from build123d import *

# Parameters (mm, degrees)
SKETCH1_W           = 124.5
SKETCH1_H           = 65.5
BOSS_EXTRUDE1_DEPTH = 1
SKETCH2_R           = 3.5
BOSS_EXTRUDE2_DEPTH = 3.5
SKETCH3_R           = 1.25
BOSS_EXTRUDE3_DEPTH = 3


with BuildPart() as part:
    # Sketch1 → Boss-Extrude1 (new body)
    with BuildSketch(Plane.XY):
        Rectangle(SKETCH1_W, SKETCH1_H)
    extrude(amount=BOSS_EXTRUDE1_DEPTH)

    # Sketch2 → Boss-Extrude2 (add)
    with BuildSketch(Plane.XY.offset(1)):
        with Locations(Location((-55.75, 24.5, 0), (0, 0, 180))):
            Circle(SKETCH2_R)
        with Locations(Location((2.25, 24.5, 0), (0, 0, 180))):
            Circle(SKETCH2_R)
        with Locations(Location((2.25, -24.5, 0), (0, 0, 180))):
            Circle(SKETCH2_R)
        with Locations(Location((-55.75, -24.5, 0), (0, 0, 180))):
            Circle(SKETCH2_R)
    extrude(amount=BOSS_EXTRUDE2_DEPTH)

    # Sketch3 → Boss-Extrude3 (add)
    with BuildSketch(Plane.XY.offset(4.5)):
        with Locations((-55.75, 24.5)):
            Circle(SKETCH3_R)
        with Locations((2.25, 24.5)):
            Circle(SKETCH3_R)
        with Locations((2.25, -24.5)):
            Circle(SKETCH3_R)
        with Locations((-55.75, -24.5)):
            Circle(SKETCH3_R)
    extrude(amount=BOSS_EXTRUDE3_DEPTH)


solid = part.part
Input: part model. Units: mm. Frame: model coordinates. A direction names the side the tool comes from. Give positions to 0.01 mm unless a question says otherwise; leave off trailing zeros. Write each loop counter-clockwise with the first axis right and the second up, starting at its lowest first coordinate (ties: lowest second). Pieces come first, ordered by that corner, then holes.
Q1. Section A-A, the plane y = 24.5. Output: boundary loops of the cut face in (x, z), plus the area to 4 significant figures.
Q2. Section B-B, the plane x = -55.75. Output: boundary loops of the cut face in (y, z), plus the area to 4 significant figures.
Q3. Set-up query: faces 1 (the face through (0.37, -27.45, 2.73)), 2 (the face through (2, 25, 7.5)). Return all of +Z, -Z, +X, -X, +Y, -Y with unobstructed straight access to the full face (end or side cutting, diameter ignored); none if empty.
Q4. Pull-direction query (X, two-part tool) for faces 3 (the face through (-56, -24, 7.5)), 4 (the face through (-52.253, 24.346, 2.726)); classes: pulls with the +X half, pulls with the -X half, needs draft (parallel to the pull), parting line crosses it, or undercut.
Q5. Section C-C, the plane x = 47. Output: boundary loops of the cut face in (y, z), plus the area to 3 significant figures.
Q6. First-contact query: P1, Ø1.5, axis at y = 22, z = 4.5, coming from the -X side. Flat tip, straight axial feed; report the tip coordinate or a pass-through.
Q7. Material intervals for probe 1 along Z at (x, y) = (-40, 30.5); probe 2 along X at (y, z) = (26.5, 4); probe 3 along X at (y, z) = (-22, 1.25), sorted ascending.
Q8. Section D-D, the plane y = -5.5. Output: boundary loops of the cut face in (x, z).
Filled in:
1. outline: (-62.25, 0) - (62.25, 0) - (62.25, 1) - (5.75, 1) - (5.75, 4.5) - (3.5, 4.5) - (3.5, 7.5) - (1, 7.5) - (1, 4.5) - (-1.25, 4.5) - (-1.25, 1) - (-52.25, 1) - (-52.25, 4.5) - (-54.5, 4.5) - (-54.5, 7.5) - (-57, 7.5) - (-57, 4.5) - (-59.25, 4.5) - (-59.25, 1) - (-62.25, 1) - close
1. area: 188.5 mm2
2. outline: (-32.75, 0) - (32.75, 0) - (32.75, 1) - (28, 1) - (28, 4.5) - (25.75, 4.5) - (25.75, 7.5) - (23.25, 7.5) - (23.25, 4.5) - (21, 4.5) - (21, 1) - (-21, 1) - (-21, 4.5) - (-23.25, 4.5) - (-23.25, 7.5) - (-25.75, 7.5) - (-25.75, 4.5) - (-28, 4.5) - (-28, 1) - (-32.75, 1) - close
2. area: 129.5 mm2
3. face 1: +Z
3. face 2: +Z, +X, -X, +Y, -Y
4. face 3: needs draft
4. face 4: undercut
5. outline: (-32.75, 0) - (32.75, 0) - (32.75, 1) - (-32.75, 1) - close
5. area: 65.5 mm2
6. P1: stops at x = -58.78
7. probe 1: z = 0 to 1
7. probe 2: x = -58.62 to -52.88, -0.62 to 5.12
7. probe 3: x = -58.2 to -53.3, -0.2 to 4.7
8. outline: (-62.25, 0) - (62.25, 0) - (62.25, 1) - (-62.25, 1) - close
